Geometry check sheet. Reference: the model listing, model coordinates, mm. A direction names the side the tool comes from. Give positions to 0.01 mm unless a question says otherwise; leave off trailing zeros. Order: outer loops, then holes, each group sorted by start corner. A loop starts at its lowest first (then second) coordinate and runs counter-clockwise, first axis right, second up. Notation, with made-up numbers: M 14.5,67 L 22.5,67 A28 ccw 22.5,99 Z; hole C -25,33.25 d10. An arc over 180 degrees is marked long. Use CSV: the item, a comma, the result in double quotes. Start each with the question number.
from build123d import *

# Parameters (mm, degrees)
F0_R     = 15.875
F1_DEPTH = 12.7
F2_R     = 3.175
F3_DEPTH = 12.7
F5_DEPTH = 5.08


with BuildPart() as f1:
    # F0 (on Top) → F1 (new body)
    with BuildSketch(Plane.XY):
        Circle(F0_R)
    extrude(amount=F1_DEPTH)

    # F2 (on face) → F3 (cut, through all)
    with BuildSketch(Plane.XY.offset(12.7)):
        Circle(F2_R)
    extrude(amount=-F3_DEPTH, mode=Mode.SUBTRACT)

    # F4 (on face) → F5 (cut)
    with BuildSketch(Plane.XY.offset(12.7)):
        with BuildLine():
            Line((6.35, 5.842), (-6.35, 5.842))
            ThreePointArc((-6.35, 5.842), (-12.192, 0), (-6.35, -5.842))
            Line((-6.35, -5.842), (6.35, -5.842))
            ThreePointArc((6.35, -5.842), (12.192, 0), (6.35, 5.842))
        make_face()
    extrude(amount=-F5_DEPTH, mode=Mode.SUBTRACT)


solid = f1.part
(1) Draft check along Y on faces 3 (the face through (0, 5.842, 10)), 4 (the face through (0, -7, 12.7)), 5 (the face through (-3.441, -15.497, 6.261)). Enter one of: +Y half, -Y half, draft (parallel to the pull), parting line (faces both ways), or undercut.
(2) Sectioned sample at B-B on x = 0. Record the cut outline in (y, z) (3 decimals), then the cut area to 3 significant figures.
(3) Go/stop test with flat-tipped pins: P1, Ø2.5, axis at x = -1.5, z = 9.5, coming from the -Y side; P2, Ø3, axis at y = -8, z = 4, coming from the +X side; P3, Ø6, axis at x = 5.5, z = 8, coming from the -Y side. Record where each tip stops, or that it passes through.
(4) Sectioned sample at D-D on z = 6. Record the cut outline in (x, y) (3 decimals).
(5) Thickness scan on line 1 (Y direction, x = 0, z = 6) (3 decimals); line 2 (Z direction, x = 3.5, y = 4.5); line 3 (X direction, y = 1.5, z = 2). Record the ranges inside material, lowest first.
(6) Sectioned sample at A-A on y = 0. Record the cut outline in (x, z) (3 decimals), then the cut area to 3 significant figures.
(7) Sectioned sample at C-C on z = 11.5. Record the cut outline in (x, y) (3 decimals).
(8) Access from +Z, -Z, +X, -X, +Y, -Y to the whole of each face (thin tool, end or side, straight path). Record for faces 1 (the face through (-12.19, 0.13, 10.2)), 2 (the face through (-0.69, -3.1, 3.86)).
Responses:
1,face 3,"undercut"
1,face 4,"draft"
1,face 5,"parting line"
2,outline,"M -15.875,0 L -3.175,0 L -3.175,7.62 L -5.842,7.62 L -5.842,12.7 L -15.875,12.7 Z; M 3.175,0 L 15.875,0 L 15.875,12.7 L 5.842,12.7 L 5.842,7.62 L 3.175,7.62 Z"
2,area,"295 mm2"
3,P1,"y = -15.87"
3,P2,"x = 14.48"
3,P3,"y = -15.68"
4,outline,"C 0,0 d31.75; hole C 0,0 d6.35"
5,line 1,"-15.875 to -3.175, 3.175 to 15.875"
5,line 2,"0 to 7.62"
5,line 3,"-15.8 to -2.8, 2.8 to 15.8"
6,outline,"M -15.875,0 L -3.175,0 L -3.175,7.62 L -12.192,7.62 L -12.192,12.7 L -15.875,12.7 Z; M 3.175,0 L 15.875,0 L 15.875,12.7 L 12.192,12.7 L 12.192,7.62 L 3.175,7.62 Z"
6,area,"231 mm2"
7,outline,"C 0,0 d31.75; hole M -6.35,-5.842 L 6.35,-5.842 A5.842 ccw 6.35,5.842 L -6.35,5.842 A5.842 ccw Z"
8,face 1,"+Z"
8,face 2,"+Z, -Z"
